Design review of the part shown in the three views and the two pictorial views. Dimensions are in mm from the part's minimum x, y and z. Give positions to 0.01 mm unless a question says otherwise; leave off trailing zeros. Order: outer loops, then holes, each group sorted by start corner. A loop starts at its lowest first (then second) coordinate and runs counter-clockwise, first axis right, second up.
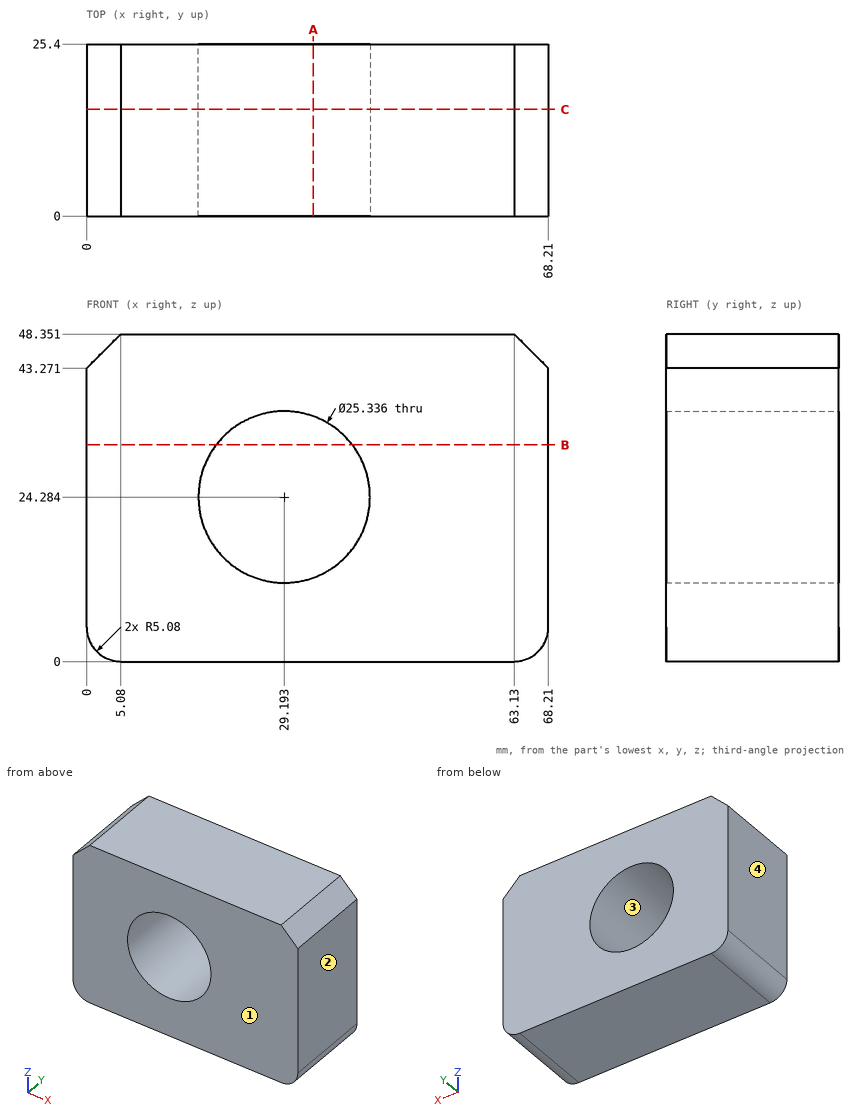
Item 1: For line 1 (X direction, y = 6, z = 23.5); line 2 (Z direction, x = 26, y = 9.25) (1 decimal); line 3 (X direction, y = 3, z = 34.5) (1 decimal), list the stretches that pass through material, from the lowest coordinate up.
Values found:
line 1: x = 0 to 16.55, 41.84 to 68.21
line 2: z = 0 to 12, 36.5 to 48.4
line 3: x = 0 to 21.7, 36.7 to 68.2
Item 2: Take a section at A-A (x = 33.5). Give the boundary of the cut face in (y, z).
Values found:
outline: (0, 0) - (25.4, 0) - (25.4, 12.37) - (0, 12.37) - close; (0, 36.2) - (25.4, 36.2) - (25.4, 48.35) - (0, 48.35) - close
Item 3: Take a section at B-B (z = 32). Give the boundary of the cut face in (x, y) (1 decimal), and give its area (3 significant figures).
Values found:
outline: (0, 0) - (19.1, 0) - (19.1, 25.4) - (0, 25.4) - close; (39.2, 0) - (68.2, 0) - (68.2, 25.4) - (39.2, 25.4) - close
area: 1,220 mm2
Item 4: Take a section at C-C (y = 15.75). Give the boundary of the cut face in (x, z) (1 decimal).
Values found:
outline: (0, 5.1) arc R5.1 ccw to (5.1, 0) - (63.1, 0) arc R5.1 ccw to (68.2, 5.1) - (68.2, 43.3) - (63.1, 48.4) - (5.1, 48.4) - (0, 43.3) - close; hole circle Ø25.3 at (29.2, 24.3)
Item 5: Draft analysis for pull direction X (two halves, no side actions). For the marked faces 1, 2, 3 and 4, state which applies: released by +X, released by -X, zero draft, split by the parting line, or undercut.
Values found:
face 1: zero draft
face 2: released by +X
face 3: undercut
face 4: released by -X
